Answer from the drawing. Dimensions are ordinates in mm from the lowest x, y and z of the part. A direction names the side the tool comes from. Round coordinates to 2 decimals unless told otherwise and drop trailing zeros. Order: outer loops, then holes, each group sorted by start corner. A loop starts at its lowest first (then second) coordinate and runs counter-clockwise, first axis right, second up. Notation, with made-up numbers: M 21,22 L 63,22 A14 cw 63,42 Z; hole C 30.25,49.5 d3. An arc over 180 degrees is marked long. Write item = value, one per line. Start each with the question number.
(1) This flat-tipped pin is pushed along its axis until it touches: pin 1 (12.5 mm diameter, centred on x = 13, y = 18, fed in from +Z). Where does it stop, or does it pass through?
(2) For a pull along X with two mould halves and no side action, classify the marked faces 1, 2 and 3 as released by +X, released by -X, zero draft, split by the parting line, or undercut.
(3) A cutting plane is placed at C-C, the plane y = 11.5. Determine the outline of the cut face in (x, z) (1 decimal).
(4) Straight lines are drawn through the part: probe 1 along Y at (x, z) = (19, 2.65); probe 2 along Y at (x, z) = (19, 0.75); probe 3 along X at (y, z) = (22.5, 2.7) (1 decimal). For each, find the intervals that lie inside material, in ascending order. Write a range as from..to.
(5) A cutting plane is placed at D-D, the plane z = 2.7. Determine the outline of the cut face in (x, y), and give its area (3 significant figures).
(6) A cutting plane is placed at A-A, the plane y = 19. Determine the outline of the cut face in (x, z).
(7) A cutting plane is placed at B-B, the plane x = 19. Determine the outline of the cut face in (y, z).
(8) Which of the six approach directions +Z, -Z, +X, -X, +Y, -Y give full straight-line access (tool end or side, diameter ignored) to the marked faces 4 and 5?
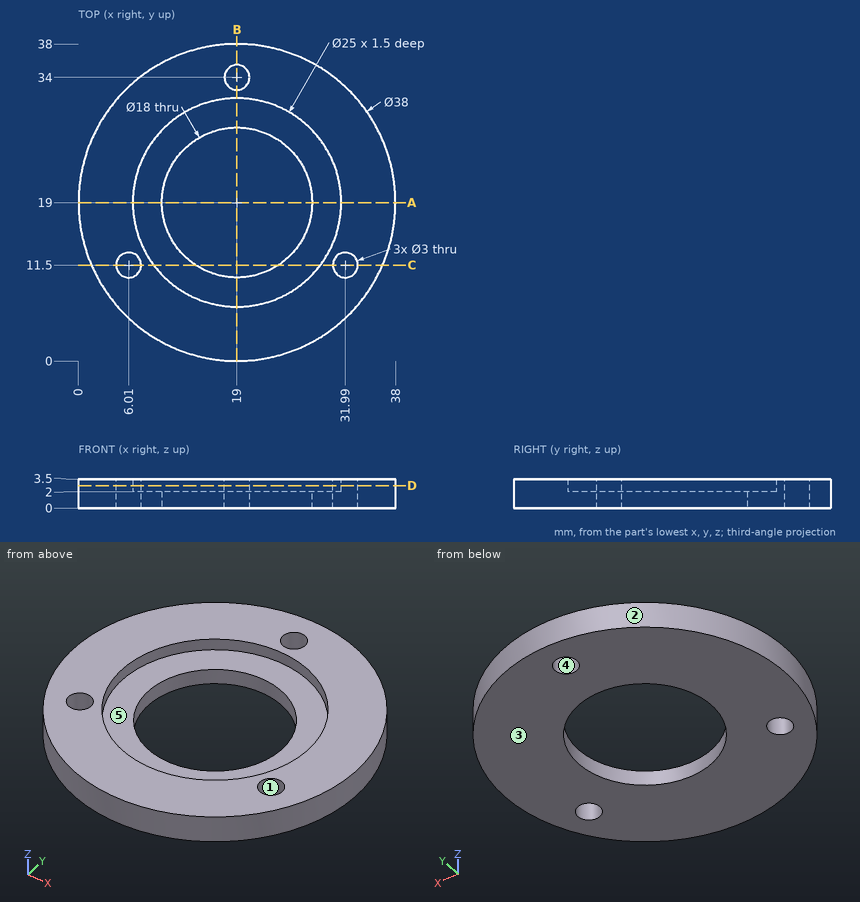
Reported:
q1.pin_1 = 2
q2.face_1 = undercut
q2.face_2 = split by the parting line
q2.face_3 = zero draft
q3.outline = M 1.5,0 L 4.5,0 L 4.5,3.5 L 1.5,3.5 Z; M 7.5,0 L 14,0 L 14,2 L 9,2 L 9,3.5 L 7.5,3.5 Z; M 24,0 L 30.5,0 L 30.5,3.5 L 29,3.5 L 29,2 L 24,2 Z; M 33.5,0 L 36.5,0 L 36.5,3.5 L 33.5,3.5 Z
q4.probe_1 = 0..6.5, 31.5..32.5, 35.5..38
q4.probe_2 = 0..10, 28..32.5, 35.5..38
q4.probe_3 = 0.3..7, 31..37.7
q5.outline = C 19,19 d38; hole C 6.01,11.5 d3; hole C 19,19 d25; hole C 19,34 d3; hole C 31.99,11.5 d3
q5.area = 622 mm²
q6.outline = M 0,0 L 10,0 L 10,2 L 6.5,2 L 6.5,3.5 L 0,3.5 Z; M 28,0 L 38,0 L 38,3.5 L 31.5,3.5 L 31.5,2 L 28,2 Z
q7.outline = M 0,0 L 10,0 L 10,2 L 6.5,2 L 6.5,3.5 L 0,3.5 Z; M 28,0 L 32.5,0 L 32.5,3.5 L 31.5,3.5 L 31.5,2 L 28,2 Z; M 35.5,0 L 38,0 L 38,3.5 L 35.5,3.5 Z
q8.face_4 = +Z, -Z
q8.face_5 = +Z
